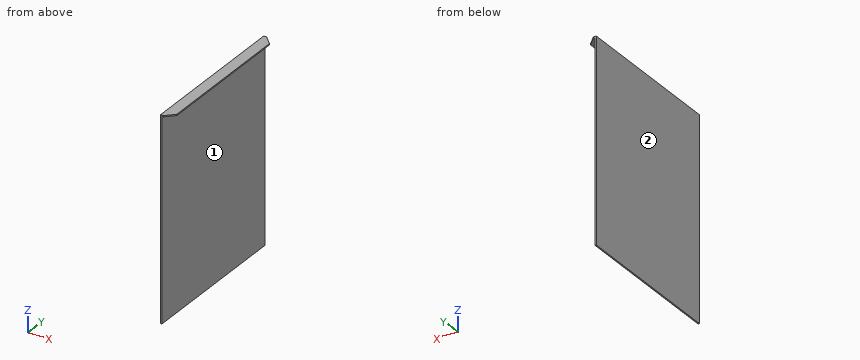
```python
from build123d import *

# Parameters (mm, degrees)
F0_W     = 195
F0_H     = 250
F1_DEPTH = 1.6
F2_W     = 195
F2_H     = 1.6
F3_DEPTH = 12
F4_SIZE  = 10


with BuildPart() as f1:
    # F0 (on Right) → F1 (new body)
    with BuildSketch(Plane.YZ):
        Rectangle(F0_W, F0_H)
    extrude(amount=F1_DEPTH)

    # F2 (on face) → F3 (join)
    with BuildSketch(Plane.YZ.offset(1.6)):
        with Locations((0, 124.2)):
            Rectangle(F2_W, F2_H)
    extrude(amount=F3_DEPTH)

    # F4
    f4_edges = [f1.edges().sort_by_distance(p)[0] for p in [
        (13.6, 97.5, 124.2),
        (13.6, -97.5, 124.2),
    ]]
    chamfer(f4_edges, length=F4_SIZE)


solid = f1.part
```
Input: part model. Units: mm. Frame: model coordinates. Face numbers are marked on the shaded views. A direction names the side the tool comes from. Give positions to 0.01 mm unless a question says otherwise; leave off trailing zeros. Order: outer loops, then holes, each group sorted by start corner. A loop starts at its lowest first (then second) coordinate and runs counter-clockwise, first axis right, second up. Notation, with made-up numbers: (-5, 76.5) - (49, 76.5) arc R10 ccw to (49, 87.5) - close; hole circle Ø1 at (60.25, 71). An arc over 180 degrees is marked (long way). Use a Markdown table: item, result.
(1) Section query C-C (y = -12). Output: boundary loops of the cut face in (x, z).
Computed values:
| item | result |
|---|---|
| outline | (0, -125) - (1.6, -125) - (1.6, 123.4) - (13.6, 123.4) - (13.6, 125) - (0, 125) - close |
(2) Pin query (flat end, axial travel): pin 1 (6 mm diameter, centred on y = -49, z = 2.5, fed in from +X); pin 2 (1 mm diameter, centred on x = 6.5, y = 28.5, fed in from -Z); pin 3 (4 mm diameter, centred on x = 5, z = 53, fed in from -Y). Return the tip coordinate at first contact, or that it passes through.
Computed values:
| item | result |
|---|---|
| pin 1 | stops at x = 1.6 |
| pin 2 | stops at z = 123.4 |
| pin 3 | passes through |
(3) Access query for the marked faces 1 and 2. Directions: +Z, -Z, +X, -X, +Y, -Y. A direction counts if a zero-diameter tool reaches every point of the face in a straight line with its end or side. Return the directions, or none.
Computed values:
| item | result |
|---|---|
| face 1 | -Z, +X, +Y, -Y |
| face 2 | +Z, -Z, -X, +Y, -Y |
(4) Section query A-A (z = 94.5). Output: boundary loops of the cut face in (x, y).
Computed values:
| item | result |
|---|---|
| outline | (0, -97.5) - (1.6, -97.5) - (1.6, 97.5) - (0, 97.5) - close |
(5) Line query: line 1 (X direction, y = -14, z = 4.5); line 2 (Z direction, x = 11.75, y = 80.5). Output: solid intervals per line, ascending. Write a range as from..to.
Computed values:
| item | result |
|---|---|
| line 1 | x = 0..1.6 |
| line 2 | z = 123.4..125 |
(6) Section query B-B (x = 8). Output: boundary loops of the cut face in (y, z), then the cut area to 3 significant figures.
Computed values:
| item | result |
|---|---|
| outline | (-93.1, 123.4) - (93.1, 123.4) - (93.1, 125) - (-93.1, 125) - close |
| area | 298 mm2 |
